Geometry check sheet. Reference: the model listing, model coordinates, mm. A direction names the side the tool comes from. Round coordinates to 2 decimals unless told otherwise and drop trailing zeros. Loops run counter-clockwise (first coordinate to the right, second up) from the corner with the lowest first, then second, coordinate; pieces in that order, holes last. Notation, with made-up numbers: M 7,-39.75 L 15,-39.75 A18 cw 15,-12.75 Z; hole C 51.25,2 d11. An arc over 180 degrees is marked long. Write item = value, one per line.
from build123d import *

# Parameters (mm, degrees)
F0_W      = 19.05
F0_H      = 387.35
F1_DEPTH  = 2057.4
F2_W      = 19.05
F2_H      = 387.35
F3_DEPTH  = 1930.4
F4_W      = 19.05
F4_H      = 387.35
F5_DEPTH  = 1930.4
F6_W      = 19.05
F6_H      = 387.35
F7_DEPTH  = 2057.4
F8_W      = 101.6
F8_H      = 101.6
F9_DEPTH  = 330.2
F10_W     = 19.05
F10_H     = 311.15
F11_DEPTH = 2025.65


with BuildPart() as f1:
    # F0 (on Front) → F1 (new body)
    with BuildSketch(Plane.XZ):
        with Locations((9.525, 193.675)):
            Rectangle(F0_W, F0_H)
    extrude(amount=F1_DEPTH)

    # F2 (on face) → F3 (join)
    with BuildSketch(Plane.YZ.offset(19.05)):
        with Locations((-2047.875, 193.675)):
            Rectangle(F2_W, F2_H)
    extrude(amount=F3_DEPTH)

    # F4 (on face) → F5 (join)
    with BuildSketch(Plane.YZ.offset(19.05)):
        with Locations((-9.525, 193.675)):
            Rectangle(F4_W, F4_H)
    extrude(amount=F5_DEPTH)

    # F6 (on Front) → F7 (join)
    with BuildSketch(Plane.XZ):
        with Locations((1958.975, 193.675)):
            Rectangle(F6_W, F6_H)
    extrude(amount=F7_DEPTH)

    # F8 (on Top) → F9 (join)
    with BuildSketch(Plane.XY):
        with Locations((69.85, -69.85)):
            Rectangle(F8_W, F8_H)
        with Locations((1898.65, -69.85)):
            Rectangle(F8_W, F8_H)
        with Locations((1898.65, -1974.85)):
            Rectangle(F8_W, F8_H)
        with Locations((69.85, -1974.85)):
            Rectangle(F8_W, F8_H)
    extrude(amount=F9_DEPTH)

    # F10 (on face) → F11 (join)
    with BuildSketch(Plane.XZ.offset(19.05)):
        with Locations((993.775, 155.575)):
            Rectangle(F10_W, F10_H)
    extrude(amount=F11_DEPTH)


solid = f1.part
(1) Material ranges on line 1 along X through (y, z) = (-1683, 62.5); line 2 along X through (y, z) = (-115, 219); line 3 along Y through (x, z) = (529.5, 127), recorded low to high. Write a range as from..to.
Result set:
line_1 = 0..19.05, 984.25..1003.3, 1949.45..1968.5
line_2 = 0..120.65, 984.25..1003.3, 1847.85..1968.5
line_3 = -2057.4..-2038.35, -19.05..0
(2) Release check for a two-part mould opening along X. For faces 1 (the flat face through (970, -2057.4, 196)), 2 (the flat face through (1003.3, -1015, 153)), 3 (the flat face through (1968.5, -1014, 191)) record: released by +X, released by -X, zero draft, split by the parting line, or undercut.
Result set:
face_1 = zero draft
face_2 = undercut
face_3 = released by +X
(3) Sectioned sample at A-A on x = 214. Record the cut outline in (y, z), then the cut area to 3 significant figures.
Result set:
outline = M -2057.4,0 L -2038.35,0 L -2038.35,387.35 L -2057.4,387.35 Z; M -19.05,0 L 0,0 L 0,387.35 L -19.05,387.35 Z
area = 14,800 mm2
(4) Sectioned sample at B-B on y = -1179. Record the cut outline in (x, z).
Result set:
outline = M 0,0 L 19.05,0 L 19.05,387.35 L 0,387.35 Z; M 984.25,0 L 1003.3,0 L 1003.3,311.15 L 984.25,311.15 Z; M 1949.45,0 L 1968.5,0 L 1968.5,387.35 L 1949.45,387.35 Z
(5) Sectioned sample at C-C on z = 30. Record the cut outline in (x, y).
Result set:
outline = M 0,-2057.4 L 1968.5,-2057.4 L 1968.5,0 L 0,0 Z; hole M 19.05,-2038.35 L 984.25,-2038.35 L 984.25,-19.05 L 120.65,-19.05 L 120.65,-120.65 L 19.05,-120.65 L 19.05,-1924.05 L 120.65,-1924.05 L 120.65,-2025.65 L 19.05,-2025.65 Z; hole M 1003.3,-2038.35 L 1949.45,-2038.35 L 1949.45,-2025.65 L 1847.85,-2025.65 L 1847.85,-1924.05 L 1949.45,-1924.05 L 1949.45,-120.65 L 1847.85,-120.65 L 1847.85,-19.05 L 1003.3,-19.05 Z
(6) Depth check by flat-ended pin: pin 1 Ø9.5 at (x, y) = (993.5, -1165) entering from +Z. Enter the tip coordinate at first touch or a pass-through.
Result set:
pin_1 = 311.15
(7) Tool access check on faces 4 (the flat face through (69, -1974, 330.2)), 5 (the flat face through (0, -1014, 191)), 6 (the flat face through (1898, -120.65, 163)). Record the directions out of +Z, -Z, +X, -X, +Y, -Y that give a thin tool (end or side, any length) a straight path to the whole face; none if there is none.
Result set:
face_4 = +Z
face_5 = +Z, -Z, -X, +Y, -Y
face_6 = +Z, -Z
